For this review, take the finished solid that the model builds, in its own axes (mm). A direction names the side the tool comes from. Round coordinates to 2 decimals unless told otherwise and drop trailing zeros. Write each loop counter-clockwise with the first axis right and the second up, starting at its lowest first coordinate (ties: lowest second). Pieces come first, ordered by that corner, then holes. Notation, with made-up numbers: (28.25, 5.25) - (70.25, 5.25) arc R23 ccw to (70.25, 28.25) - close; hole circle Ø7 at (-23.5, 11.25). An arc over 180 degrees is marked (long way). One line per item, written item: value. Start each with the question number.
Q1. For probe 1 along X at (y, z) = (-35.5, 12.5); probe 2 along Y at (x, z) = (7, 7); probe 3 along Y at (x, z) = (12.5, 15.5), list the stretches that pass through material, from the lowest coordinate up.
Q2. Add section A-A on z = -1.25. Write out the cut boundary in (x, y), and give its area (3 significant figures).
Q3. Add section B-B on y = -166.5. Write out the cut boundary in (x, z), and give its area (3 significant figures).
Q4. Tool access review of faces 4 (the face through (10.426, -99, 7)), 5 (the face through (4, -200, 4)), 6 (the face through (0.426, -99, 10)): name each direction out of +Z, -Z, +X, -X, +Y, -Y from which nothing blocks a thin tool from reaching the whole face with its end or side.
Q5. Clearance check with flat-ended pins moving along their axes: pin 1 Ø8 at (x, y) = (-2.5, -89.5) entering from +Z; pin 2 Ø12 at (x, z) = (-3, 16) entering from -Y; pin 3 Ø2.5 at (x, y) = (3.5, -74.5) entering from +Z. State where each tip first meets the part, or that it passes through.
Q6. Add section C-C on z = 9.25. Write out the cut boundary in (x, y), and give its area (3 significant figures).
Q7. Mouldability with a two-part tool opening along X and no side actions: class faces 1 (the face through (12, 9.25, 10)), 2 (the face through (14.676, -99, 7)), 3 (the face through (-2.65, -98.6, 3.56)) as +X half, -X half, draft (parallel to the pull), parting line (faces both ways), or undercut.
Q8. Add section D-D on x = 2.75. Write out the cut boundary in (y, z), and give its area (3 significant figures).
```python
from build123d import *

# Parameters (mm, degrees)
F0_W      = 5
F0_H      = 12
F1_DEPTH  = 200
F2_R      = 2
F3_W      = 14.25
F3_H      = 9.25
F4_DEPTH  = 30
F6_DEPTH  = 9.25
F7_W      = 14.25
F7_H      = 9.25
F8_DEPTH  = 30
F9_W      = 9.25
F9_H      = 4.25
F10_DEPTH = 25


with BuildPart() as f1:
    # F0 (on Front) → F1 (new body)
    with BuildSketch(Plane.XZ):
        Polygon((0.426156, 14.766954), (-6.573844, 14.766954), (0.426156, -5.233046), (0.426156, 6.766954), align=None)
        with Locations((2.926156, 0.766954)):
            Rectangle(F0_W, F0_H)
        Polygon((5.426156, 6.766954), (5.426156, -5.233046), (10.426156, -5.233046), (10.426156, 19.766954), (14.676156, 19.766954), (14.676156, -5.233046), (19.676156, -5.233046), (19.676156, 24.766954), (5.426156, 24.766954), align=None)
    extrude(amount=F1_DEPTH)

    # F2
    f2_edges = [f1.edges().sort_by_distance(p)[0] for p in [
        (-6.573844, -100, 14.766954),
        (0.426156, -100, 14.766954),
    ]]
    fillet(f2_edges, radius=F2_R)

    # F3 (on face) → F4 (join)
    with BuildSketch(Plane.XY.offset(24.766954)):
        with Locations((12.551156, 4.625)):
            Rectangle(F3_W, F3_H)
    extrude(amount=-F4_DEPTH)

    # F5 (on face) → F6 (cut)
    with BuildSketch(Plane(origin=(5.426156, 0, 0), x_dir=(0, -1, 0), z_dir=(-1, 0, 0))):
        Polygon((-4.25, -5.233046), (0, -5.233046), (0, 6.766954), (0, 19.047581), (-4.25, 19.047581), align=None)
    extrude(amount=-F6_DEPTH, mode=Mode.SUBTRACT)

    # F7 (on face) → F8 (join)
    with BuildSketch(Plane.XY.offset(24.766954)):
        with Locations((12.551156, -204.625)):
            Rectangle(F7_W, F7_H)
    extrude(amount=-F8_DEPTH)

    # F9 (on face) → F10 (cut)
    with BuildSketch(Plane(origin=(0, 0, -5.233046), x_dir=(1, 0, 0), z_dir=(0, 0, -1))):
        with Locations((10.051156, 202.125)):
            Rectangle(F9_W, F9_H)
    extrude(amount=-F10_DEPTH, mode=Mode.SUBTRACT)


solid = f1.part
```
Result set:
1. probe 1: x = -5.74 to 0.43, 5.43 to 10.43, 14.68 to 19.68
1. probe 2: y = -209.25 to -204.25, -200 to 0, 4.25 to 9.25
1. probe 3: y = -209.25 to -204.25, 4.25 to 9.25
2. outline: (-0.97, -200) - (10.43, -200) - (10.43, 0) - (-0.97, 0) - close; (5.43, -209.25) - (19.68, -209.25) - (19.68, 9.25) - (5.43, 9.25) - (5.43, 4.25) - (14.68, 4.25) - (14.68, -204.25) - (5.43, -204.25) - close
2. area: 3,460 mm^2
3. outline: (-5.64, 12.11) - (0.43, -5.23) - (10.43, -5.23) - (10.43, 19.77) - (14.68, 19.77) - (14.68, -5.23) - (19.68, -5.23) - (19.68, 24.77) - (5.43, 24.77) - (5.43, 6.77) - (0.43, 6.77) - (0.43, 12.77) arc R2 ccw to (-1.57, 14.77) - (-3.75, 14.77) arc R2 ccw to start
3. area: 449 mm^2
4. face 4: -Z
4. face 5: -Z, -X
4. face 6: +Z, +Y, -Y
5. pin 1: stops at z = 14.77
5. pin 2: stops at y = -200
5. pin 3: stops at z = 6.77
6. outline: (-4.64, -200) - (0.43, -200) - (0.43, 0) - (-4.64, 0) - close; (5.43, -209.25) - (19.68, -209.25) - (19.68, 9.25) - (5.43, 9.25) - (5.43, 4.25) - (14.68, 4.25) - (14.68, -204.25) - (5.43, -204.25) - close; (5.43, -200) - (10.43, -200) - (10.43, 0) - (5.43, 0) - close
6. area: 3,200 mm^2
7. face 1: draft
7. face 2: undercut
7. face 3: -X half
8. outline: (-200, -5.23) - (0, -5.23) - (0, 6.77) - (-200, 6.77) - close
8. area: 2,400 mm^2
